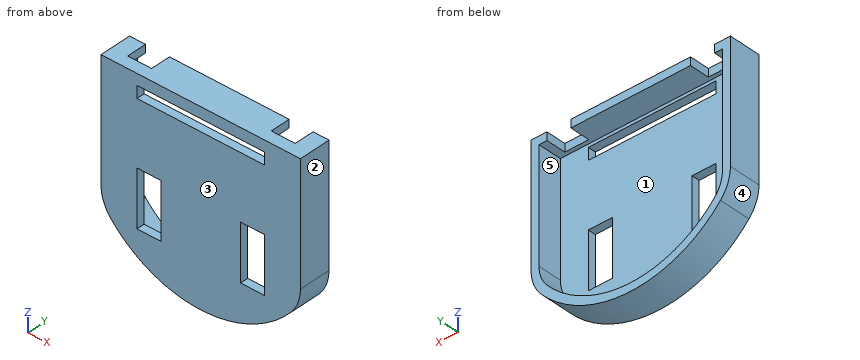
```python
from build123d import *

# Parameters (mm, degrees)
BOSS_EXTRUDE1_DEPTH = 40
SHELL1_T            = -10
SKETCH2_W           = 30
SKETCH2_H           = 70
SKETCH2_W_2         = 160
SKETCH2_H_2         = 15
CUT_EXTRUDE1_DEPTH  = 198.547462651
CUT_EXTRUDE2_REACH  = 270.167
SKETCH3_W           = 30
SKETCH3_H           = 50


with BuildPart() as part:
    # Sketch1 → Boss-Extrude1 (new body)
    with BuildSketch(Plane(origin=(0, 0, 0), x_dir=(1, 0, 0), z_dir=(0, 1, 0))):
        with BuildLine():
            Line((125, 66.143782777), (125, -83.856217223))
            Line((125, -83.856217223), (-125, -83.856217223))
            Line((-125, -83.856217223), (-125, 66.143782777))
            ThreePointArc((-125, 66.143782777), (-121.770717335, 83.821452306), (-112.5, 99.215674165))
            ThreePointArc((-112.5, 99.215674165), (0, 150), (112.5, 99.215674165))
            ThreePointArc((112.5, 99.215674165), (121.770717335, 83.821452306), (125, 66.143782777))
        make_face()
    extrude(amount=BOSS_EXTRUDE1_DEPTH)

    # Shell1
    shell1_openings = [part.faces().sort_by_distance(p)[0] for p in [
        (0, 40, -23.901312182),
    ]]
    offset(amount=SHELL1_T, openings=shell1_openings, kind=Kind.INTERSECTION)

    # Sketch2 → Cut-Extrude1 (cut, through all)
    with BuildSketch(Plane(origin=(0, 10, 0), x_dir=(1, 0, 0), z_dir=(0, 1, 0))):
        with Locations((-65, 60)):
            Rectangle(SKETCH2_W, SKETCH2_H)
        with Locations((65, 60)):
            Rectangle(SKETCH2_W, SKETCH2_H)
        with Locations((0, -62.5)):
            Rectangle(SKETCH2_W_2, SKETCH2_H_2)
    extrude(amount=-CUT_EXTRUDE1_DEPTH, mode=Mode.SUBTRACT)

    # Sketch3 → Cut-Extrude2 (cut, up to next)
    with BuildSketch(Plane.XY.offset(83.856217223), mode=Mode.PRIVATE) as cut_extrude2_sk1:
        with Locations((-90, 40)):
            Rectangle(SKETCH3_W, SKETCH3_H)
    cut_extrude2_tool1 = extrude(cut_extrude2_sk1.sketch, amount=-CUT_EXTRUDE2_REACH, mode=Mode.PRIVATE) & part.part
    # Sketch3 → Cut-Extrude2 (cut, up to next)
    with BuildSketch(Plane.XY.offset(83.856217223), mode=Mode.PRIVATE) as cut_extrude2_sk2:
        with Locations((90, 40)):
            Rectangle(SKETCH3_W, SKETCH3_H)
    cut_extrude2_tool2 = extrude(cut_extrude2_sk2.sketch, amount=-CUT_EXTRUDE2_REACH, mode=Mode.PRIVATE) & part.part
    add(cut_extrude2_tool1.solids().sort_by_distance((-90, 40, 83.856217))[0], mode=Mode.SUBTRACT)
    add(cut_extrude2_tool2.solids().sort_by_distance((90, 40, 83.856217))[0], mode=Mode.SUBTRACT)


solid = part.part
```
Source: CAD feature listing. Evaluate the final solid. Frame: model axes, mm. Face numbers are marked on the shaded views. A direction names the side the tool comes from. Round coordinates to 2 decimals unless told otherwise and drop trailing zeros. Loops run counter-clockwise (first coordinate to the right, second up) from the corner with the lowest first, then second, coordinate; pieces in that order, holes last.
1. Access query for the marked faces 1 and 2. Directions: +Z, -Z, +X, -X, +Y, -Y. A direction counts if a zero-diameter tool reaches every point of the face in a straight line with its end or side. Return the directions, or none.
2. Ray query, L1, parallel to X at y = 3, z = -36.5; L2, parallel to X at y = 18.5, z = -29.5; L3, parallel to Y at x = 77, z = -103. Return the intervals inside material, ascending.
3. Section query D-D on z = 64.5. Output: boundary loops of the cut face in (x, y).
4. Section query A-A on y = 19. Output: boundary loops of the cut face in (x, z), and give its area (3 significant figures).
5. Section query C-C on x = -29.5. Output: boundary loops of the cut face in (y, z).
6. Section query B-B on z = -40. Output: boundary loops of the cut face in (x, y), and give its area (3 significant figures).
7. Mould query, pull axis Z, two halves, no side actions, for the marked faces 3, 4 and 5. Classes: released by +Z, released by -Z, zero draft, split by the parting line, or undercut.
8. Contact query for flat-ended pins moving along their axis: pin 1 (8 mm diameter, centred on x = -69.5, y = 4.5, fed in from -Z); pin 2 (5 mm diameter, centred on x = -43.5, z = -78.5, fed in from -Y); pin 3 (3 mm diameter, centred on x = -86.5, z = 77.5, fed in from +Y); pin 4 (5 mm diameter, centred on y = 20.5, z = -120, fed in from +X). Output: stop coordinate, or through.
Answers below:
1. face 1: +Y
1. face 2: +Z, -Z, +X, +Y, -Y
2. L1: x = -125 to -80, -50 to 50, 80 to 125
2. L2: x = -125 to -115, 115 to 125
2. L3: y = 0 to 10
3. outline: (-125, 0) - (-80, 0) - (-80, 10) - (-115, 10) - (-115, 40) - (-125, 40) - close; (80, 0) - (125, 0) - (125, 40) - (115, 40) - (115, 10) - (80, 10) - close
4. outline: (-125, -66.14) arc R50 ccw to (-112.5, -99.22) arc R150 ccw to (112.5, -99.22) arc R50 ccw to (125, -66.14) - (125, 83.86) - (105, 83.86) - (105, 73.86) - (115, 73.86) - (115, -66.14) arc R40 cw to (105, -92.6) arc R140 cw to (-105, -92.6) arc R40 cw to (-115, -66.14) - (-115, 73.86) - (-105, 73.86) - (-105, 83.86) - (-125, 83.86) - close; (-75, 73.86) - (75, 73.86) - (75, 83.86) - (-75, 83.86) - close
4. area: 7,810 mm2
5. outline: (0, -147.07) - (40, -147.07) - (40, -136.86) - (10, -136.86) - (10, 55) - (0, 55) - close; (0, 70) - (10, 70) - (10, 73.86) - (40, 73.86) - (40, 83.86) - (0, 83.86) - close
6. outline: (-125, 0) - (-80, 0) - (-80, 10) - (-115, 10) - (-115, 40) - (-125, 40) - close; (-50, 0) - (50, 0) - (50, 10) - (-50, 10) - close; (80, 0) - (125, 0) - (125, 40) - (115, 40) - (115, 10) - (80, 10) - close
6. area: 2,500 mm2
7. face 3: zero draft
7. face 4: released by -Z
7. face 5: undercut
8. pin 1: stops at z = -134.94
8. pin 2: stops at y = 0
8. pin 3: stops at y = 15
8. pin 4: stops at x = 93.24
